The model under review builds one solid part; all positions refer to its coordinate system, in mm. A direction names the side the tool comes from. Coordinates: 2 decimals unless noted, no trailing zeros. Loops run counter-clockwise (first coordinate to the right, second up) from the corner with the lowest first, then second, coordinate; pieces in that order, holes last. Notation, with made-up numbers: (68.5, 30) - (87.5, 30) arc R21 ccw to (87.5, 56) - close; hole circle Ø4 at (89, -14). An arc over 180 degrees is marked (long way). One line per item, written item: value. Start each with the question number.
1. To check wall thickness, follow line 1 (Z direction, x = -5.25, y = 3.5); line 2 (Z direction, x = -7.25, y = 5.25); line 3 (Z direction, x = -1, y = 1.5). State the ranges of each line that lie inside material, in increasing order.
2. We need section A-A, the plane z = 21. Give the boundary of the cut face in (x, y), then the cut area to 3 significant figures.
3. Mouldability with a two-part tool opening along X and no side actions: class faces 5 (the face through (-1.68, 5.18, -1.97)), 6 (the face through (-2.13, -1.24, -7.7)), 7 (the face through (-3, 2.44, 18)) as +X half, -X half, draft (parallel to the pull), parting line (faces both ways), or undercut.
4. We need section B-B, the plane x = -5.5. Give the boundary of the cut face in (y, z).
5. For faces 1 (the face through (-4, 4, -8.937)), 2 (the face through (-7, 5, 3)), 3 (the face through (-3, 4.84, 19)), 4 (the face through (-5, 3, 0.5)), list the 3-axis set-ups (+Z, -Z, +X, -X, +Y, -Y) from which the entire face can be reached by the end or side of a thin tool; tool diameter is ignored.
6. We need section D-D, the plane y = 1. Give the boundary of the cut face in (x, z).
7. Insertion check: P1, Ø3, axis at y = 3, z = 4, coming from the +X side; P2, Ø3, axis at x = -7.5, z = 0, coming from the +Y side; P3, Ø2.5, axis at x = -8, y = 4, coming from the +Z side. Each pin has a flat end and moves straight along its axis. Give the tip position at first contact, or say it passes through.
8. We need section C-C, the plane x = -3.5. Give the boundary of the cut face in (y, z), then the cut area to 3 significant figures.
Autodesk Inventor part; units mm, degrees
ref_plane "Arbeitsebene1" through (-10.5829, -3.5471, -5.9368) normal (0, 0, -1) x (0, 1, 0)
ref_plane "YZ Plane" through (0, 0, 0) normal (1, 0, 0) x (0, 1, 0)
ref_plane "XZ Plane" through (0, 0, 0) normal (0, 1, 0) x (-1, 0, 0)
sketch "Skizze1" plane through (0, 0, 0) normal (0, 0, 1) x (1, 0, 0)
  line L0 (0, 0) -> (-5.0357, 8.6396)
  line L1 (-5.0357, 8.6396) -> (-9.3555, 6.1217)
  line L2 (-4.3198, -2.5178) -> (-9.3555, 6.1217)
  line L3 (0, 0) -> (-4.3198, -2.5178)
  line L4 (0, 0) -> (0, 8.6396)
  line L5 (0, 8.6396) -> (-5.0357, 8.6396)
extrude "Extrusion1" add sketch "Skizze1" along normal blind 3
sketch "Skizze2" plane through (0, 0, 3) normal (0, 0, 1) x (1, 0, 0)
  line L0 (0, 8.6396) -> (-5.0357, 8.6396)
  line L1 (0, 0) -> (0, 8.6396)
  line L2 (-4.3198, -2.5178) -> (0, 0)
  line L3 (-9.3555, 6.1217) -> (-4.3198, -2.5178)
  line L4 (-5.0357, 8.6396) -> (-9.3555, 6.1217)
  line L5 (0, 0) -> (-5.0357, 8.6396)
  line L6 (0, 0) -> (-4.3198, -2.5178)
  line L7 (-9.3555, 6.1217) -> (-4.3198, -2.5178)
  line L8 (-5.0357, 8.6396) -> (-9.3555, 6.1217)
ref_plane "Arbeitsebene1" through (-10.5829, -3.5471, -5.9368) normal (0, 0, -1) x (0, 1, 0)
extrude "Extrusion2" add sketch "Skizze2" against normal up to surface (8.9368 mm away) contours L1 L5 L0
sketch "Skizze3" plane through (0, 8.6396, -5.9368) normal (0, 0, -1) x (-1, 0, 0)
  line L0 (6.3089, -7.7448) -> (1.9891, -5.2269)
  line L1 (0, -8.6396) -> (5.0357, 0)
  line L2 (0, -8.6396) -> (4.3198, -11.1574)
  line L3 (9.3555, -2.5178) -> (4.3198, -11.1574)
  line L4 (5.0357, 0) -> (9.3555, -2.5178)
  line L5 (0, -8.6396) -> (0, 0)
  line L6 (5.0357, 0) -> (0, -8.6396)
  line L7 (0, 0) -> (5.0357, 0)
extrude "Extrusion3" add sketch "Skizze3" along normal blind 3
sketch "Skizze4" plane through (-5.0357, 8.6396, -5.9368) normal (-0.8639552, -0.5035686, 0) x (0, 0, 1)
  circle A0 centre (2.9684, -5) radius 1.05
  point P0 (5.9368, -10)
extrude "Extrusion4" cut sketch "Skizze4" against normal through all
sketch "Skizze6" plane through (0, 0, 3) normal (0, 0, 1) x (1, 0, 0)
  line L0 (-5.0357, 8.6396) -> (-9.3555, 6.1217)
  line L1 (-9.3555, 6.1217) -> (-4.3198, -2.5178)
  line L2 (-4.3198, -2.5178) -> (0, 0)
  line L3 (0, 0) -> (0, 8.6396)
  line L4 (0, 8.6396) -> (-5.0357, 8.6396)
extrude "Extrusion5" add sketch "Skizze6" along normal blind 30
sketch "Skizze7" plane through (0, 0, 33) normal (0, 0, 1) x (1, 0, 0)
  line L0 (0, 8.6396) -> (0, 0)
  line L1 (0, 8.6396) -> (-6, 8.6396)
  line L2 (-6, 8.6396) -> (-6, -6.275)
  line L3 (-6, -6.275) -> (0, -6.275)
  line L4 (0, -6.275) -> (0, 8.6396)
  line L5 (-4.3198, -2.5178) -> (0, 0)
  line L6 (0, 0) -> (0, 8.6396)
  line L7 (0, 8.6396) -> (-5.0357, 8.6396)
  line L8 (-5.0357, 8.6396) -> (-9.3555, 6.1217)
  line L9 (-9.3555, 6.1217) -> (-4.3198, -2.5178)
  point P0 (-6, 0.3649)
  point P1 (-6, 8.0775)
  dimension "d10" = 6
extrude "Extrusion6" cut sketch "Skizze7" against normal blind 30 contours L2 L9 L8
sketch "Skizze8" plane through (-6, 0.3649, 33) normal (-1, 0, 0) x (0, 0, 1)
  line L0 (-3.2, 3.2747) -> (-25.8, 3.2747) construction
  line L1 (-3.2, 4.4747) -> (-25.8, 4.4747)
  line L2 (-25.8, 2.0747) -> (-3.2, 2.0747)
  arc A0 (-3.2, 2.0747) -> (-3.2, 4.4747) centre (-3.2, 3.2747) ccw
  arc A1 (-25.8, 4.4747) -> (-25.8, 2.0747) centre (-25.8, 3.2747) ccw
  line L3 (0, 7.7126) -> (0, 0)
  line L4 (-33, 8.2747) -> (0, 8.2747)
  point P0 (-33, -0.3649)
  point P1 (-14.5, 3.2747)
  dimension "d13" = 2.4
  dimension "d14" = 25
  dimension "d15" = 2
  dimension "d16" = 5
extrude "Extrusion7" cut sketch "Skizze8" against normal blind 30
ref_plane "Arbeitsebene2" through (0, 8.6396, -8.9368) normal (-0.8639552, -0.5035686, 0) x (0, 0, 1)
sketch "Skizze9" plane through (0, 8.6396, -8.9368) normal (-0.8639552, -0.5035686, 0) x (0, 0, 1)
  circle A0 centre (5.9684, -2.4642) radius 1.05
  circle A1 centre (5.9684, -2.4642) radius 1.05
  circle A2 centre (5.9684, -2.4642) radius 2.2
  point P0 (8.9368, -7.4642)
  dimension "d19" = 4.4
extrude "Extrusion8" cut sketch "Skizze9" along normal blind 2
sketch "Skizze10" plane through (0, 0, 0) normal (0, 0, -1) x (-1, 0, 0)
  line L0 (5.0357, 8.6396) -> (0, 0)
  line L1 (4.3198, -2.5178) -> (0, 0)
  line L2 (9.3555, 6.1217) -> (4.3198, -2.5178)
  line L3 (5.0357, 8.6396) -> (9.3555, 6.1217)
extrude "Extrusion9" cut sketch "Skizze10" along normal blind 6.5 and the other way blind 0.5
properties part number "Slider"
Findings below:
1. line 1: -8.94 to -6.5, 0.5 to 6.01, 30.99 to 33
1. line 2: -8.94 to -6.5, 0.5 to 3
1. line 3: -8.94 to -6.5, 0.5 to 33
2. outline: (-6, 0.36) - (-4.32, -2.52) - (0, 0) - (0, 2.44) - (-6, 2.44) - close; (-6, 4.84) - (0, 4.84) - (0, 8.64) - (-5.04, 8.64) - (-6, 8.08) - close
2. area: 44.4 mm2
3. face 5: undercut
3. face 6: +X half
3. face 7: draft
4. outline: (-0.49, -8.94) - (8.37, -8.94) - (8.37, -6.5) - (-0.49, -6.5) - close; (-0.49, 0.5) - (8.37, 0.5) - (8.37, 33) - (-0.49, 33) - close; hole (2.44, 7.2) arc R1.2 ccw to (4.84, 7.2) - (4.84, 29.8) arc R1.2 ccw to (2.44, 29.8) - close
5. face 1: -Z, +X, -X, +Y, -Y
5. face 2: +Z, -X, +Y, -Y
5. face 3: +X, -X
5. face 4: -X, -Y
6. outline: (-6.37, -8.94) - (0, -8.94) - (0, 33) - (-6, 33) - (-6, 3) - (-6.37, 3) - (-6.37, 0.5) - (-0.58, 0.5) - (-0.58, -6.5) - (-6.37, -6.5) - close
7. P1: x = 0
7. P2: y = 8.03
7. P3: z = 3
8. outline: (-2.04, -8.94) - (8.64, -8.94) - (8.64, 33) - (-2.04, 33) - (-2.04, 0.5) - (6, 0.5) - (6, -6.5) - (-2.04, -6.5) - close; hole (2.44, 7.2) arc R1.2 ccw to (4.84, 7.2) - (4.84, 29.8) arc R1.2 ccw to (2.44, 29.8) - close
8. area: 333 mm2
